from build123d import *

# Parameters (mm, degrees)
CROQUIS1_W              = 23
CROQUIS1_H              = 30.3
SALIENTE_EXTRUIR2_DEPTH = 10
CROQUIS3_W              = 7
CROQUIS3_H              = 19
CORTAR_EXTRUIR1_DEPTH   = 40.333064971
CROQUIS4_W              = 11
CROQUIS4_H              = 23
SALIENTE_EXTRUIR3_DEPTH = 3
CROQUIS5_R              = 1.5
CORTAR_EXTRUIR3_DEPTH   = 40.333064971
CROQUIS6_R              = 1.5
CORTAR_EXTRUIR4_DEPTH   = 42.688007868
NERVIO10_REACH          = 38.622
CROQUIS23_WALL_W        = 82.243156676
CROQUIS23_WALL_H        = 7


with BuildPart() as part:
    # Croquis1 → Saliente-Extruir2 (new body)
    with BuildSketch(Plane(origin=(0, 0, 0), x_dir=(0, 0, -1), z_dir=(1, 0, 0))):
        with Locations((-11.5, -15.15)):
            Rectangle(CROQUIS1_W, CROQUIS1_H)
    extrude(amount=SALIENTE_EXTRUIR2_DEPTH)

    # Croquis3 → Cortar-Extruir1 (cut, through all)
    with BuildSketch(Plane(origin=(0, 0, 0), x_dir=(1, 0, 0), z_dir=(0, 1, 0))):
        with Locations((6.5, -12.5)):
            Rectangle(CROQUIS3_W, CROQUIS3_H)
    extrude(amount=-CORTAR_EXTRUIR1_DEPTH, mode=Mode.SUBTRACT)

    # Croquis4 → Saliente-Extruir3 (add)
    with BuildSketch(Plane.XZ.offset(30.3)):
        with Locations((-2.5, 11.5)):
            Rectangle(CROQUIS4_W, CROQUIS4_H)
    extrude(amount=SALIENTE_EXTRUIR3_DEPTH)

    # Croquis5 → Cortar-Extruir3 (cut, through all)
    with BuildSketch(Plane(origin=(0, -30.3, 0), x_dir=(1, 0, 0), z_dir=(0, 1, 0))):
        with Locations(Location((-4, -4, 0), (0, 0, 270))):
            Circle(CROQUIS5_R)
        with Locations(Location((-4, -19, 0), (0, 0, 270))):
            Circle(CROQUIS5_R)
    extrude(amount=-CORTAR_EXTRUIR3_DEPTH, mode=Mode.SUBTRACT)

    # Croquis6 → Cortar-Extruir4 (cut, through all)
    with BuildSketch(Plane.XY.offset(23)):
        with Locations(Location((6, -5, 0), (0, 0, 270))):
            Circle(CROQUIS6_R)
    extrude(amount=-CORTAR_EXTRUIR4_DEPTH, mode=Mode.SUBTRACT)

    # Croquis23 wall → Nervio10 (add, up to next)
    with BuildSketch(Plane(origin=(-2.474873734, -27.825126266, 11.5), x_dir=(0.707106781187, 0.707106781187, 0), z_dir=(-0.707106781187, 0.707106781187, 0)), mode=Mode.PRIVATE) as nervio10_sk1:
        Rectangle(CROQUIS23_WALL_W, CROQUIS23_WALL_H)
    nervio10_tool1 = extrude(nervio10_sk1.sketch, amount=-NERVIO10_REACH, mode=Mode.PRIVATE) - part.part
    add(nervio10_tool1.solids().sort_by_distance((-2.474873734, -27.825126266, 11.5))[0])


solid = part.part
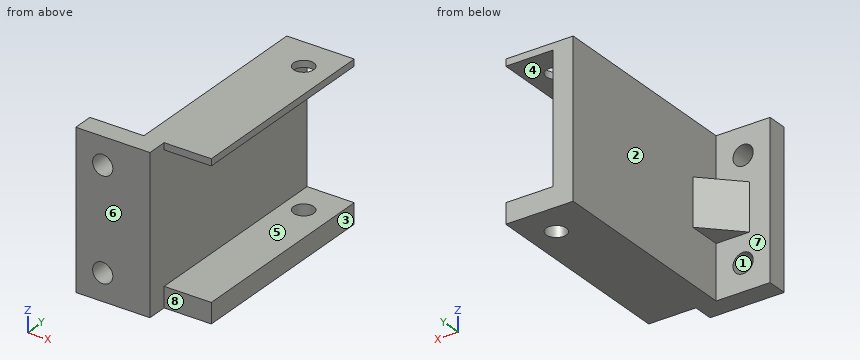
The model under review builds one solid part; all positions refer to its coordinate system, in mm. Face numbers are marked on the shaded views. A direction names the side the tool comes from. Coordinates: 2 decimals unless noted, no trailing zeros. Write each loop counter-clockwise with the first axis right and the second up, starting at its lowest first coordinate (ties: lowest second). Pieces come first, ordered by that corner, then holes. Notation, with made-up numbers: (46, 6) -> (56, 6) arc R8 cw to (56, 11) -> close; hole circle Ø4 at (-28, 78.25). An arc over 180 degrees is marked (long way). Answer in a Markdown table with one row per item.
1. We need section C-C, the plane x = 6. State the section outline as (y, z) points, and give its area (3 significant figures).
Answers below:
| item | result |
|---|---|
| outline | (-30.3, 0) -> (-6.5, 0) -> (-6.5, 3) -> (-30.3, 3) -> close; (-30.3, 22) -> (-6.5, 22) -> (-6.5, 23) -> (-30.3, 23) -> close; (-3.5, 0) -> (0, 0) -> (0, 3) -> (-3.5, 3) -> close; (-3.5, 22) -> (0, 22) -> (0, 23) -> (-3.5, 23) -> close |
| area | 109 mm^2 |
2. Draft analysis for pull direction X (two halves, no side actions). For the marked faces 1, 2, 3 and 4, state which applies: +X half, -X half, draft (parallel to the pull), parting line (faces both ways), or undercut.
Answers below:
| item | result |
|---|---|
| face 1 | undercut |
| face 2 | -X half |
| face 3 | +X half |
| face 4 | draft |
3. Clearance check with flat-ended pins moving along their axes: pin 1 Ø1.5 at (x, y) = (-1.5, -26.5) entering from -Z; pin 2 Ø1 at (y, z) = (-15.5, 5) entering from +X; pin 3 Ø1.5 at (y, z) = (-25.5, 5.5) entering from -X; pin 4 Ø3.5 at (x, z) = (-4, 4) entering from -Y. State where each tip first meets the part, or that it passes through.
Answers below:
| item | result |
|---|---|
| pin 1 | stops at z = 8 |
| pin 2 | stops at x = 3 |
| pin 3 | stops at x = 0 |
| pin 4 | stops at y = -33.3 |
4. For the marked faces 5, 6, 7 and 8, list the 3-axis set-ups (+Z, -Z, +X, -X, +Y, -Y) from which the entire face can be reached by the end or side of a thin tool; tool diameter is ignored.
Answers below:
| item | result |
|---|---|
| face 5 | +X, +Y, -Y |
| face 6 | +Z, -Z, +X, -X, -Y |
| face 7 | -X, +Y |
| face 8 | +Z, -Z, +X, -Y |
5. Wall thickness on probe 1 along Z at (x, y) = (7.5, -21); probe 2 along X at (y, z) = (-31.75, 19); probe 3 along Y at (x, z) = (-7, 11.25): over which ranges is each line inside the solid? List them lowest first. Write a range as [from, to].
Answers below:
| item | result |
|---|---|
| probe 1 | z = [0, 3], [22, 23] |
| probe 2 | x = [-8, -5.5], [-2.5, 3] |
| probe 3 | y = [-33.3, -30.3] |
6. We need section D-D, the plane x = -4. State the section outline as (y, z) points.
Answers below:
| item | result |
|---|---|
| outline | (-33.3, 0) -> (-30.3, 0) -> (-30.3, 2.5) -> (-33.3, 2.5) -> close; (-33.3, 5.5) -> (-30.3, 5.5) -> (-30.3, 8) -> (-29.35, 8) -> (-29.35, 15) -> (-30.3, 15) -> (-30.3, 17.5) -> (-33.3, 17.5) -> close; (-33.3, 20.5) -> (-30.3, 20.5) -> (-30.3, 23) -> (-33.3, 23) -> close |
7. We need section B-B, the plane z = 19. State the section outline as (x, y) points, and give its area (3 significant figures).
Answers below:
| item | result |
|---|---|
| outline | (-8, -33.3) -> (-5.5, -33.3) -> (-5.5, -30.3) -> (-8, -30.3) -> close; (-2.5, -33.3) -> (3, -33.3) -> (3, 0) -> (0, 0) -> (0, -30.3) -> (-2.5, -30.3) -> close |
| area | 115 mm^2 |
8. We need section A-A, the plane y = -5. State the section outline as (x, z) points.
Answers below:
| item | result |
|---|---|
| outline | (0, 0) -> (4.5, 0) -> (4.5, 3) -> (3, 3) -> (3, 22) -> (4.5, 22) -> (4.5, 23) -> (0, 23) -> close; (7.5, 0) -> (10, 0) -> (10, 3) -> (7.5, 3) -> close; (7.5, 22) -> (10, 22) -> (10, 23) -> (7.5, 23) -> close |
